```python
from build123d import *

# Parameters (mm, degrees)
ESQUISSE7_R                  = 16
ENL_V_MAT_EXTRU_4_DEPTH      = 31
ENL_V_MAT_EXTRU_4_DEPTH_BACK = 20.75582071
ENL_V_MAT_EXTRU_5_DEPTH      = 18.457623262
ENL_V_MAT_EXTRU_5_DEPTH_BACK = 18.457623262


with BuildPart() as part:
    # Esquisse6 → Révolution3 (revolve)
    with BuildSketch(Plane.XY, mode=Mode.PRIVATE) as r_volution3_sk:
        Polygon((30.254629316, 29.023433988), (49.837753266, -5.976566012), (51.58312395, -5), (32, 30), align=None)
    revolve(r_volution3_sk.sketch.rotate(Axis((16, 30, 0), (0.422618262, -0.906307787, 0)), 180), axis=Axis((16, 30, 0), (0.422618262, -0.906307787, 0)))  # turned: the seam where the file's is

    # Esquisse7 → Enlèv. mat.-Extru.4 (cut, two sides)
    with BuildSketch(Plane(origin=(0, 0, 0), x_dir=(1, 0, 0), z_dir=(0, 1, 0))) as enl_v_mat_extru_4_sk:
        with Locations((16, 0)):
            Circle(ESQUISSE7_R)
    extrude(amount=ENL_V_MAT_EXTRU_4_DEPTH, mode=Mode.SUBTRACT)
    extrude(enl_v_mat_extru_4_sk.sketch, amount=-ENL_V_MAT_EXTRU_4_DEPTH_BACK, mode=Mode.SUBTRACT)

    # Esquisse8 → Enlèv. mat.-Extru.5 (cut, two sides)
    with BuildSketch(Plane.XY) as enl_v_mat_extru_5_sk:
        with BuildLine():
            Line((0, 0), (35, 0))
            ThreePointArc((35, 0), (56.213203436, -8.786796564), (65, -30))
            Line((65, -30), (0, -30))
            Line((0, -30), (0, 0))
        make_face()
    extrude(amount=ENL_V_MAT_EXTRU_5_DEPTH, mode=Mode.SUBTRACT)
    extrude(enl_v_mat_extru_5_sk.sketch, amount=-ENL_V_MAT_EXTRU_5_DEPTH_BACK, mode=Mode.SUBTRACT)


solid = part.part
```
The listing builds one solid part. Answer for the finished solid, in the listing's coordinates (mm). Coordinates: 2 decimals unless noted, no trailing zeros. Use one line per item in the form item = value. Start each with the question number.
Item 1: The mould has two halves that part along Z. Classify faces 1 (the face through (39.473, 16.631, -0.44)), 2 (the face through (29, 0, 15)), 3 (the face through (31.94, 26.04, -1.37)): released by +Z, released by -Z, zero draft, split by the parting line, or undercut.
Item 2: Consider L1, parallel to Z at x = 34.5, y = 15; L2, parallel to Z at x = 28, y = 22; L3, parallel to Y at x = 34.5, z = -11. Determine where each line is inside the solid, lowest interval first. Write a range as [from, to].
Item 3: Flat-ended cylindrical pins translate along their axes: pin 1 Ø2.5 at (x, z) = (28.5, -15) entering from -Y; pin 2 Ø4 at (y, z) = (23.5, -9.5) entering from +X; pin 3 Ø6 at (x, y) = (26.5, 8) entering from -Z. Find the tip coordinate at first contact, or state that the pin passes through.
Answer key:
q1.face_1 = split by the parting line
q1.face_2 = zero draft
q1.face_3 = undercut
q2.L1 = [-11.58, -8.7], [8.7, 11.58]
q2.L2 = [-12.89, -10.58], [10.58, 12.89]
q2.L3 = [10.39, 16.18]
q3.pin_1 = 0
q3.pin_2 = 33.75
q3.pin_3 = -16.02
